Input: dimensioned drawing with shaded views. Units: mm. Origin: part minimum x, y, z. A direction names the side the tool comes from. Coordinates: 2 decimals unless noted, no trailing zeros. Order: outer loops, then holes, each group sorted by start corner. A loop starts at its lowest first (then second) coordinate and runs counter-clockwise, first axis right, second up. Notation, with made-up numbers: (51.5, -24.5) -> (97.5, -24.5) arc R35 ccw to (97.5, 10.5) -> close; hole circle Ø9 at (66.25, 29). An arc over 180 degrees is marked (long way). Answer as CSV lines item,"result".
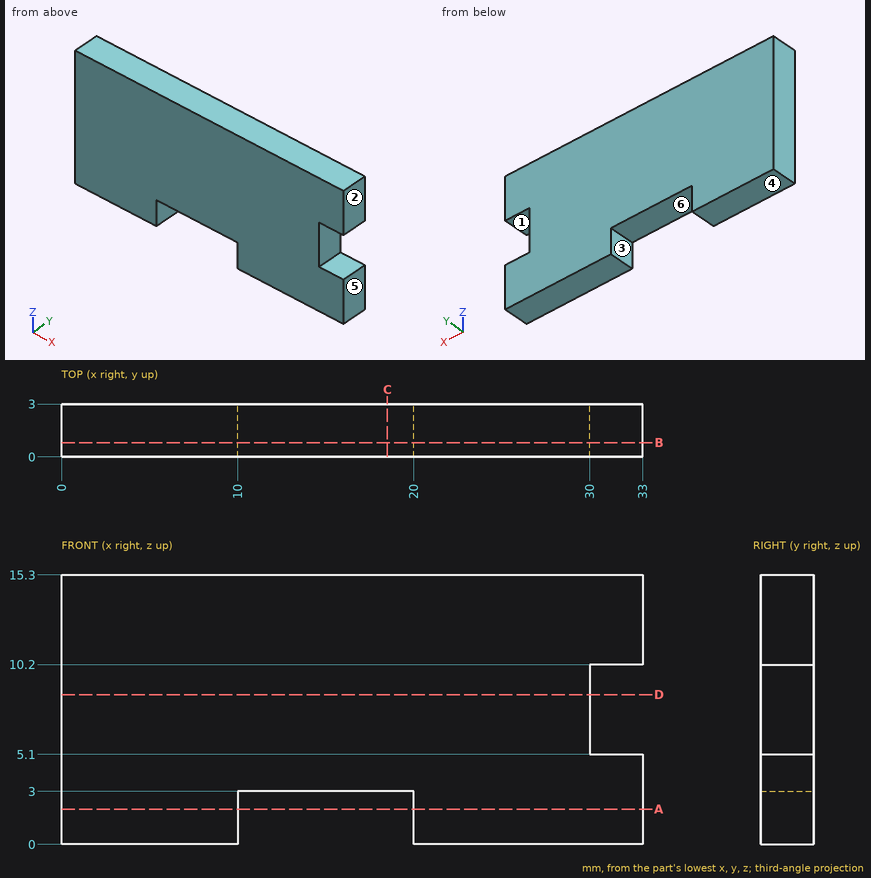
1. Cut plane B-B (y = 0.8). Return the cut outline in (x, z).
Findings:
outline,"(0, 0) -> (10, 0) -> (10, 3) -> (20, 3) -> (20, 0) -> (33, 0) -> (33, 5.1) -> (30, 5.1) -> (30, 10.2) -> (33, 10.2) -> (33, 15.3) -> (0, 15.3) -> close"
2. Cut plane C-C (x = 18.5). Return the cut outline in (y, z), plus the area to 3 significant figures.
Findings:
outline,"(0, 3) -> (3, 3) -> (3, 15.3) -> (0, 15.3) -> close"
area,"36.9 mm2"
3. Cut plane A-A (z = 2). Return the cut outline in (x, y).
Findings:
outline,"(0, 0) -> (10, 0) -> (10, 3) -> (0, 3) -> close; (20, 0) -> (33, 0) -> (33, 3) -> (20, 3) -> close"
4. Mould query, pull axis X, two halves, no side actions, for the marked faces 3, 4, 5 and 6. Classes: released by +X, released by -X, zero draft, split by the parting line, or undercut.
Findings:
face 3,"undercut"
face 4,"zero draft"
face 5,"released by +X"
face 6,"undercut"
5. Reachability of the marked faces 1 and 2 from +Z, -Z, +X, -X, +Y, -Y: full face, straight path, thin tool, end or side. Return the list, or none.
Findings:
face 1,"+X, +Y, -Y"
face 2,"+Z, -Z, +X, +Y, -Y"
6. Ray query, line 1 along Z through (x, y) = (31, 0.7); line 2 along X through (y, z) = (2.85, 2); line 3 along X through (y, z) = (0.7, 6.75). Return the intervals inside material, ascending.
Findings:
line 1,"z = 0 to 5.1, 10.2 to 15.3"
line 2,"x = 0 to 10, 20 to 33"
line 3,"x = 0 to 30"
7. Contact query for flat-ended pins moving along their axis: pin 1 (0.9 mm diameter, centred on y = 2, z = 9, fed in from +X); pin 2 (0.9 mm diameter, centred on x = 16, y = 1, fed in from -Z). Output: stop coordinate, or through.
Findings:
pin 1,"stops at x = 30"
pin 2,"stops at z = 3"
8. Cut plane D-D (z = 8.5). Return the cut outline in (x, y).
Findings:
outline,"(0, 0) -> (30, 0) -> (30, 3) -> (0, 3) -> close"
